Check sheet for the modelled part. Datum: model origin and axes. Units: mm. Face numbers are marked on the shaded views. Round coordinates to 2 decimals unless told otherwise and drop trailing zeros. Order: outer loops, then holes, each group sorted by start corner. A loop starts at its lowest first (then second) coordinate and runs counter-clockwise, first axis right, second up. Notation, with made-up numbers: (45.25, -25) -> (75.25, -25) arc R27 ccw to (75.25, 11) -> close; hole circle Ø5 at (84.25, 6.25). An arc over 180 degrees is marked (long way). Use CSV: the item, a comma, the result in double quotes.
```python
from build123d import *

# Parameters (mm, degrees)
BOSS_EXTRUDE1_DEPTH = 3.175


with BuildPart() as part:
    # Sketch1 → Boss-Extrude1 (new body)
    with BuildSketch(Plane(origin=(0, 24.05298106, 51.338092747), x_dir=(1, 0, 0), z_dir=(0, 0.42426395071815903, 0.9055385690963249))):
        with BuildLine():
            Line((-223.489586571, 437.581228051), (-204.439586571, 437.581228051))
            Line((-204.439586571, 437.581228051), (-204.439586571, 424.881228051))
            ThreePointArc((-204.439586571, 424.881228051), (-213.964586571, 415.356228051), (-223.489586571, 424.881228051))
            Line((-223.489586571, 424.881228051), (-223.489586571, 437.581228051))
        make_face()
        with BuildLine():
            Line((-210.789586571, 422.341228051), (-210.789586571, 429.961228051))
            ThreePointArc((-210.789586571, 429.961228051), (-213.964586571, 433.136228051), (-217.139586571, 429.961228051))
            Line((-217.139586571, 429.961228051), (-217.139586571, 422.341228051))
            ThreePointArc((-217.139586571, 422.341228051), (-213.964586571, 419.166228051), (-210.789586571, 422.341228051))
        make_face(mode=Mode.SUBTRACT)
    extrude(amount=BOSS_EXTRUDE1_DEPTH)


solid = part.part
```
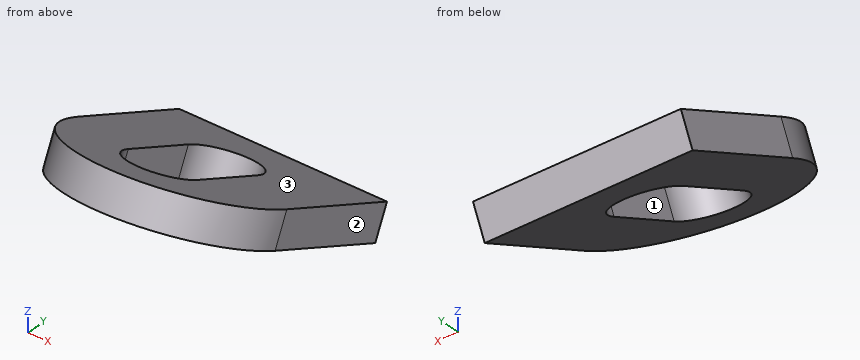
Q1. Scan lines: L1, parallel to Y at x = -222, z = -128; L2, parallel to Y at x = -210, z = -130.75; L3, parallel to Z at x = -218.75, y = 402.25. Record each from-to range of solid material in increasing order.
Result sheet:
L1,"y = 406.83 to 414.31"
L2,"y = 412.7 to 420.18"
L3,"z = -125.86 to -123.49"
Q2. Sectioned sample at D-D, the plane x = -209. Enter the section's corners in (y, z).
Result sheet:
outline,"(401.44, -125.47) -> (420.3, -134.31) -> (421.65, -131.44) -> (402.79, -122.6) -> close"
Q3. Mould release check, pull along X, two halves, no side actions. Record for the marked faces 1, 2 and 3: pulls with the +X half, pulls with the -X half, needs draft (parallel to the pull), parting line crosses it, or undercut.
Result sheet:
face 1,"undercut"
face 2,"pulls with the +X half"
face 3,"needs draft"
Q4. Go/stop test with flat-tipped pins: pin 1 (6 mm diameter, centred on x = -208, y = 402.5, fed in from -Z); pin 2 (1.5 mm diameter, centred on x = -219.5, y = 417.5, fed in from +Z); pin 3 (2 mm diameter, centred on x = -221, y = 414.5, fed in from -Z). Record where each tip stops, or that it passes through.
Result sheet:
pin 1,"stops at z = -127.38"
pin 2,"stops at z = -129.14"
pin 3,"stops at z = -132.06"
Q5. Sectioned sample at B-B, the plane x = -213. Enter the section's corners in (y, z), then the cut area to 3 significant figures.
Result sheet:
outline,"(400.22, -124.9) -> (403.76, -126.56) -> (405.11, -123.69) -> (401.57, -122.03) -> close; (416.14, -132.36) -> (420.3, -134.31) -> (421.65, -131.44) -> (417.49, -129.49) -> close"
area,"27.0 mm^2"
Q6. Sectioned sample at C-C, the plane z = -133. Enter the section's corners in (x, y).
Result sheet:
outline,"(-223.49, 417.5) -> (-204.44, 417.5) -> (-204.44, 420.91) -> (-223.49, 420.91) -> close"
Q7. Sectioned sample at A-A, the plane x = -215. Enter the section's corners in (y, z), then the cut area to 3 significant figures.
Result sheet:
outline,"(400.23, -124.91) -> (403.78, -126.57) -> (405.13, -123.7) -> (401.57, -122.03) -> close; (416.12, -132.35) -> (420.3, -134.31) -> (421.65, -131.44) -> (417.46, -129.48) -> close"
area,"27.1 mm^2"
